The model under review builds one solid part; all positions refer to its coordinate system, in mm. Face numbers are marked on the shaded views. A direction names the side the tool comes from. Coordinates: 2 decimals unless noted, no trailing zeros. Order: outer loops, then holes, each group sorted by start corner. A loop starts at its lowest first (then second) coordinate and runs counter-clockwise, first axis right, second up.
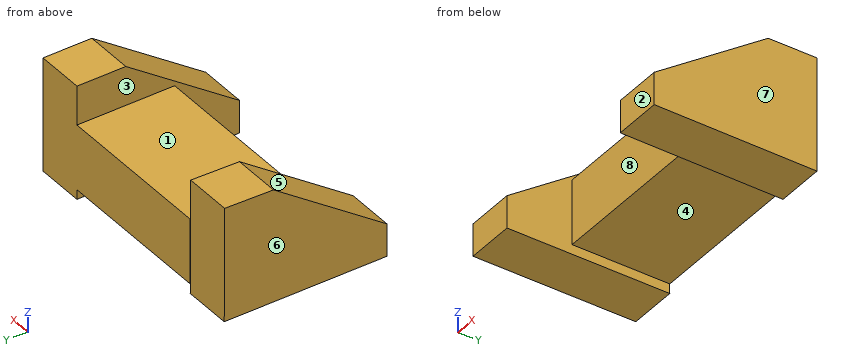
from build123d import *

# Parameters (mm, degrees)
F0_W     = 63.5
F0_H     = 38.1
F1_DEPTH = 25.4
F3_DEPTH = 19.05
F5_DEPTH = 19.05


with BuildPart() as f1:
    # F0 (on Top) → F1 (new body)
    with BuildSketch(Plane.XY):
        with Locations((-1.108171, 18.795629)):
            Rectangle(F0_W, F0_H)
    extrude(amount=F1_DEPTH)

    # F2 (on face) → F3 (join)
    with BuildSketch(Plane.YZ.offset(30.641829)):
        Polygon((37.845629, -3.775676), (37.845629, 0), (37.845629, 40.674324), (18.795629, 40.674324), (-25.653121, 9.322739), (-25.653121, -3.377261), align=None)
    extrude(amount=F3_DEPTH)

    # F4 (on face) → F5 (join)
    with BuildSketch(Plane(origin=(-32.858171, 0, 0), x_dir=(0, -1, 0), z_dir=(-1, 0, 0))):
        Polygon((-18.634845, 40.211677), (-37.67904, 40.681904), (-37.845629, -3.767784), (25.654371, -3.767784), (25.654371, 8.932216), align=None)
    extrude(amount=F5_DEPTH)


solid = f1.part
(1) Insertion check: pin 1 Ø11.5 at (x, y) = (4, 17.5) entering from -Z; pin 2 Ø21 at (x, y) = (40.5, 26) entering from +Z; pin 3 Ø4 at (x, z) = (15.5, 19) entering from -Y. Each pin has a flat end and moves straight along its axis. Give the tip position at first contact, or say it passes through.
(2) Consider section C-C (x = 41). Give the boundary of the cut face in (y, z).
(3) Consider section D-D (z = 13.5). Give the boundary of the cut face in (x, y).
(4) The part is to be moulded in two halves that separate along X. For the marked faces 5, 6, 7 and 8, say which applies: +X half, -X half, draft (parallel to the pull), parting line (faces both ways), or undercut.
(5) Consider section B-B (z = 33). Give the boundary of the cut face in (x, y).
(6) Wall thickness on line 1 (X direction, y = -10.5, z = -0.5); line 2 (Y direction, x = 16.5, z = 18.5); line 3 (Z direction, x = -28, y = 2): over which ranges is each line inside the solid? List them lowest first.
(7) Consider section A-A (y = -10.5). Give the boundary of the cut face in (x, z).
(8) Tool access review of the marked faces 1, 2, 3 and 4: name each direction out of +Z, -Z, +X, -X, +Y, -Y from which nothing blocks a thin tool from reaching the whole face with its end or side.
Findings:
1. pin 1: stops at z = 0
1. pin 2: stops at z = 40.67
1. pin 3: stops at y = -0.25
2. outline: (-25.65, -3.38) - (37.85, -3.78) - (37.85, 40.67) - (18.8, 40.67) - (-25.65, 9.32) - close
3. outline: (-51.91, -19.19) - (-32.86, -19.19) - (-32.86, -0.25) - (30.64, -0.25) - (30.64, -19.73) - (49.69, -19.73) - (49.69, 37.85) - (-32.86, 37.85) - (-32.86, 37.78) - (-51.91, 37.78) - close
4. face 5: draft
4. face 6: -X half
4. face 7: +X half
4. face 8: undercut
5. outline: (-51.91, 8.42) - (-32.86, 8.42) - (-32.86, 37.71) - (-51.91, 37.71) - close; (30.64, 7.92) - (49.69, 7.92) - (49.69, 37.85) - (30.64, 37.85) - close
6. line 1: x = -51.91 to -32.86, 30.64 to 49.69
6. line 2: y = -0.25 to 37.85
6. line 3: z = 0 to 25.4
7. outline: (-51.91, -3.77) - (-32.86, -3.77) - (-32.86, 19.64) - (-51.91, 19.64) - close; (30.64, -3.47) - (49.69, -3.47) - (49.69, 20.01) - (30.64, 20.01) - close
8. face 1: +Z, +Y, -Y
8. face 2: +Z, -Z, +X, -X, -Y
8. face 3: -Y
8. face 4: -Z, +Y, -Y
